```python
from build123d import *

# Parameters (mm, degrees)
F0_W     = 15.3924
F0_H     = 8.001
F1_DEPTH = 15.6718
F3_DEPTH = 7.493
F5_DEPTH = 7.9502
F7_DEPTH = 7.62


with BuildPart() as f1:
    # F0 (on Front) → F1 (new body)
    with BuildSketch(Plane.XZ):
        with Locations((23.4442, 4.0005)):
            Rectangle(F0_W, F0_H)
        Polygon((0, 16.1036), (0, 0), (15.748, 0), (15.748, 8.001), (15.748, 16.1036), align=None)
    extrude(amount=F1_DEPTH)

    # F2 (on face) → F3 (join)
    with BuildSketch(Plane(origin=(0, 0, 0), x_dir=(-1, 0, 0), z_dir=(0, 1, 0))):
        Polygon((-31.1404, 16.1036), (-31.1404, 8.001), (-15.748, 8.001), (-23.113546893, 16.1036), align=None)
    extrude(amount=-F3_DEPTH)

    # F4 (on face) → F5 (join)
    with BuildSketch(Plane(origin=(0, 0, 0), x_dir=(-1, 0, 0), z_dir=(0, 1, 0))):
        Polygon((-7.366, 0), (0, 0), (0, 7.7724), align=None)
    extrude(amount=F5_DEPTH)

    # F6 (on face) → F7 (join)
    with BuildSketch(Plane(origin=(0, 7.9502, 0), x_dir=(-1, 0, 0), z_dir=(0, 1, 0))):
        Polygon((-7.366, 0), (0, 0), (0, 7.7724), align=None)
        Polygon((-7.366, 16.163635999), (-7.366, 0), (0, 7.7724), (0, 16.163635999), align=None)
    extrude(amount=F7_DEPTH)


solid = f1.part
```
Input: part model. Units: mm. Frame: model coordinates. A direction names the side the tool comes from. Round coordinates to 2 decimals unless told otherwise and drop trailing zeros. Loops run counter-clockwise (first coordinate to the right, second up) from the corner with the lowest first, then second, coordinate; pieces in that order, holes last. Notation, with made-up numbers: (48.25, 15) -> (82.25, 15) arc R19 ccw to (82.25, 25) -> close; hole circle Ø11 at (18, -4.75). An arc over 180 degrees is marked (long way). Write each question's results on one line, items separated by ' | '.
1. Ray query, line 1 (Y direction, x = 7, z = 6.75); line 2 (X direction, y = 8, z = 4); line 3 (Y direction, x = 12.5, z = 6.75). Return the intervals inside material, ascending. Write a range as from..to.
Geometry results:
line 1: -15.67..0, 7.95..15.57 | line 2: 0..7.37 | line 3: -15.67..0
2. Section A-A (z = 10.5). Return loops of the section in (x, y).
Geometry results:
outline: (0, -15.67) -> (15.75, -15.67) -> (15.75, 0) -> (0, 0) -> close; (0, 7.95) -> (7.37, 7.95) -> (7.37, 15.57) -> (0, 15.57) -> close; (18.02, -7.49) -> (31.14, -7.49) -> (31.14, 0) -> (18.02, 0) -> close
3. Section B-B (y = -6.5). Return loops of the section in (x, z), and give its area (3 significant figures).
Geometry results:
outline: (0, 0) -> (31.14, 0) -> (31.14, 16.1) -> (23.11, 16.1) -> (15.75, 8) -> (15.75, 16.1) -> (0, 16.1) -> close | area: 472 mm2
4. Section D-D (z = 5). Return loops of the section in (x, y).
Geometry results:
outline: (0, -15.67) -> (31.14, -15.67) -> (31.14, 0) -> (2.63, 0) -> (2.63, 7.95) -> (7.37, 7.95) -> (7.37, 15.57) -> (0, 15.57) -> close
5. Set-up query: faces 1 (the face through (8, -8, 16.104)), 2 (the face through (3.63, 3.92, 3.94)), 3 (the face through (23, -12, 8.001)). Return all of +Z, -Z, +X, -X, +Y, -Y with unobstructed straight access to the full face (end or side cutting, diameter ignored); none if empty.
Geometry results:
face 1: +Z, +X, -X, -Y | face 2: +Z, +X | face 3: +Z, +X, -Y
6. Mould query, pull axis Y, two halves, no side actions, for faces 4 (the face through (19.379, -3.694, 11.996)), 5 (the face through (4, 15.57, 8)), 6 (the face through (16, 0, 6)). Classes: +Y half, -Y half, draft (parallel to the pull), parting line (faces both ways), or undercut.
Geometry results:
face 4: draft | face 5: +Y half | face 6: undercut
7. First-contact query: P1, Ø17, axis at x = 6.5, y = -11.5, coming from the +Z side; P2, Ø4, axis at y = 11, z = 11.5, coming from the +X side; P3, Ø6, axis at x = 20, z = 4.5, coming from the +Y side; P4, Ø4, axis at x = 18, y = 3.5, coming from the +Z side. Flat tips, straight axial feed; report the tip coordinate or a pass-through.
Geometry results:
P1: z = 16.1 | P2: x = 7.37 | P3: y = 0 | P4: through
8. Section C-C (x = 2.5). Return loops of the section in (y, z), and give its area (3 significant figures).
Geometry results:
outline: (-15.67, 0) -> (15.57, 0) -> (15.57, 16.16) -> (7.95, 16.16) -> (7.95, 5.13) -> (0, 5.13) -> (0, 16.1) -> (-15.67, 16.1) -> close | area: 416 mm2
